Geometry: final body of the model. Coordinates: model frame, mm. A direction names the side the tool comes from. Give positions to 0.01 mm unless a question says otherwise; leave off trailing zeros. Write each loop counter-clockwise with the first axis right and the second up, starting at its lowest first coordinate (ties: lowest second). Pieces come first, ordered by that corner, then holes. Notation, with made-up numbers: M 9,-14.75 L 49,-14.75 A14 cw 49,7.25 Z; hole C -35.5,46 d1. An arc over 180 degrees is marked long. Use one line per item in the form item = value. Start each with the question number.
Item 1: Pull-direction query (X, two-part tool) for faces 1 (the cylindrical face through (-9.36, 8.94, -10.21)), 2 (the cylindrical face through (-0.135, 2.267, -6.437)), 3 (the conical face through (9.24, 1.76, -9.3)); classes: released by +X, released by -X, zero draft, split by the parting line, or undercut.
Item 2: Section query B-B on y = 10.5. Return loops of the section in (x, z), then the cut area to 3 significant figures.
Item 3: Access query for faces 4 (the flat face through (0, 15.2, -12)), 5 (the flat face through (0, 3.5, -12)), 6 (the flat face through (0, 3.5, 12)). Directions: +Z, -Z, +X, -X, +Y, -Y. A direction counts if a zero-diameter tool reaches every point of the face in a straight line with its end or side. Return the directions, or none.
Item 4: Contact query for flat-ended pins moving along their axis: P1, Ø1, axis at y = 8, z = 1.5, coming from the -X side; P2, Ø4.5, axis at x = -11.5, z = 2.5, coming from the -Y side; P3, Ø4, axis at x = -11, z = -10, coming from the -Y side. Output: stop coordinate, or through.
Item 5: Section query A-A on x = 0. Return loops of the section in (y, z).
Item 6: Material intervals for line 1 along X through (y, z) = (11.75, 0); line 2 along Y through (x, z) = (6.5, -2.5); line 3 along Y through (x, z) = (0.25, -1), sorted ascending. Write a range as from..to.
from build123d import *

# Parameters (mm, degrees)
SKETCH2_R                                     = 11.35
CUT_EXTRUDE1_DEPTH                            = 14
SKETCH3_R                                     = 7.414246795
CUT_EXTRUDE2_DEPTH                            = 35.581714822
CIRPATTERN1_COUNT                             = 4
CSK_FOR_M3_COUNTERSUNK_FLAT_HEAD1_D           = 3.4
CSK_FOR_M3_COUNTERSUNK_FLAT_HEAD1_DEPTH       = 2.5
CSK_FOR_M3_COUNTERSUNK_FLAT_HEAD1_CSINK_D     = 4
CSK_FOR_M3_COUNTERSUNK_FLAT_HEAD1_CSINK_ANGLE = 90
CSK_FOR_M3_COUNTERSUNK_FLAT_HEAD3_D           = 3.4
CSK_FOR_M3_COUNTERSUNK_FLAT_HEAD3_DEPTH       = 2.5
CSK_FOR_M3_COUNTERSUNK_FLAT_HEAD3_CSINK_D     = 4
CSK_FOR_M3_COUNTERSUNK_FLAT_HEAD3_CSINK_ANGLE = 90
CUT_EXTRUDE4_DEPTH                            = 2.5
CIRPATTERN2_COUNT                             = 3


with BuildPart() as part:
    # Sketch1 → Revolve1 (revolve)
    with BuildSketch(Plane.XY, mode=Mode.PRIVATE) as revolve1_sk:
        Polygon((0, 0), (-1, 0), (-1, 1), (-12.35, 1), (-13.85, 2.5), (-13.85, 15.2), (-11.35, 17.7), (-2.5, 17.7), (-2.5, 31), (-1.5, 32), (0, 32), align=None)
    revolve(revolve1_sk.sketch.rotate(Axis((0, 41.020495061, 0), (0, -1, 0)), 270), axis=Axis((0, 41.020495061, 0), (0, -1, 0)))

    # Sketch2 → Cut-Extrude1 (cut)
    with BuildSketch(Plane(origin=(0, 3.5, 0), x_dir=(1, 0, 0), z_dir=(0, 1, 0))):
        with Locations(Location((0, 0, 0), (0, 0, 90))):
            Circle(SKETCH2_R)
    extrude(amount=CUT_EXTRUDE1_DEPTH, mode=Mode.SUBTRACT)

    # Sketch3 → Cut-Extrude2 (cut, through all)
    with BuildSketch(Plane(origin=(0, 3.5, 0), x_dir=(1, 0, 0), z_dir=(0, 1, 0))):
        with Locations((0, -13.85)):
            Circle(SKETCH3_R)
    cut_extrude2 = extrude(amount=-CUT_EXTRUDE2_DEPTH, mode=Mode.SUBTRACT)

    # CirPattern1: Cut-Extrude2 ×4 about axis
    cirpattern1_axis = Axis((0, 0, 0), (0, 1, 0))
    for i in range(1, CIRPATTERN1_COUNT):
        add(cut_extrude2.rotate(cirpattern1_axis, i * 360 / CIRPATTERN1_COUNT), mode=Mode.SUBTRACT)

    # CSK for M3 Countersunk Flat Head1
    with Locations(Plane(origin=(0, 1, 0), x_dir=(-1, 0, 0), z_dir=(0, -1, 0))):
        with Locations((5.656854249, -5.656854249), (-5.656854249, 5.656854249)):
            CounterSinkHole(CSK_FOR_M3_COUNTERSUNK_FLAT_HEAD1_D / 2, CSK_FOR_M3_COUNTERSUNK_FLAT_HEAD1_CSINK_D / 2, depth=CSK_FOR_M3_COUNTERSUNK_FLAT_HEAD1_DEPTH, counter_sink_angle=CSK_FOR_M3_COUNTERSUNK_FLAT_HEAD1_CSINK_ANGLE)

    # CSK for M3 Countersunk Flat Head3
    with Locations(Plane(origin=(0, 1, 0), x_dir=(-1, 0, 0), z_dir=(0, -1, 0))):
        with Locations((6.717514421, 6.717514421), (-6.717514421, -6.717514421)):
            CounterSinkHole(CSK_FOR_M3_COUNTERSUNK_FLAT_HEAD3_D / 2, CSK_FOR_M3_COUNTERSUNK_FLAT_HEAD3_CSINK_D / 2, depth=CSK_FOR_M3_COUNTERSUNK_FLAT_HEAD3_DEPTH, counter_sink_angle=CSK_FOR_M3_COUNTERSUNK_FLAT_HEAD3_CSINK_ANGLE)

    # Sketch16 → Cut-Extrude4 (cut)
    with BuildSketch(Plane(origin=(0, 17.7, 0), x_dir=(1, 0, 0), z_dir=(0, 1, 0))):
        with BuildLine():
            Line((-4.79581004, 12.993179213), (-8.169414432, 7.879287267))
            Line((-8.169414432, 7.879287267), (-1.815909947, 1.718275607))
            ThreePointArc((-1.815909947, 1.718275607), (0, 2.5), (1.815909947, 1.718275607))
            Line((1.815909947, 1.718275607), (8.169414432, 7.879287267))
            Line((8.169414432, 7.879287267), (4.79581004, 12.993179213))
            Line((4.79581004, 12.993179213), (0, 16.897060704))
            Line((0, 16.897060704), (-4.79581004, 12.993179213))
        make_face()
    cut_extrude4 = extrude(amount=-CUT_EXTRUDE4_DEPTH, mode=Mode.SUBTRACT)

    # CirPattern2: Cut-Extrude4 ×3 about axis
    cirpattern2_axis = Axis((0, 0, 0), (0, 1, 0))
    for i in range(1, CIRPATTERN2_COUNT):
        add(cut_extrude4.rotate(cirpattern2_axis, i * 360 / CIRPATTERN2_COUNT), mode=Mode.SUBTRACT)


solid = part.part
Answer sheet:
q1.face_1 = split by the parting line
q1.face_2 = undercut
q1.face_3 = released by +X
q2.outline = C 0,0 d27.7; hole C 0,0 d22.7
q2.area = 198 mm2
q3.face_4 = +Y
q3.face_5 = -Z, -Y
q3.face_6 = +Z, -Y
q4.P1 = -13.81
q4.P2 = 3.5
q4.P3 = 1.52
q5.outline = M 0,-1 L 1,-1 L 1,-6.44 L 3.5,-6.44 L 3.5,6.44 L 1,6.44 L 1,1 L 0,1 Z; M 3.5,-13.85 L 15.2,-13.85 L 15.2,-11.35 L 3.5,-11.35 Z; M 3.5,11.35 L 17.5,11.35 L 17.5,-2.5 L 31,-2.5 L 32,-1.5 L 32,1.5 L 31,2.5 L 17.7,2.5 L 17.7,11.35 L 15.2,13.85 L 3.5,13.85 Z
q6.line_1 = -13.85..-11.35, 11.35..13.85
q6.line_2 = 1..3.5, 17.5..17.7
q6.line_3 = 1..3.5, 17.5..32
